Read the model definition and answer for the solid it produces. Units are mm, in the model's axes. Face numbers are marked on the shaded views. A direction names the side the tool comes from. Coordinates: 2 decimals unless noted, no trailing zeros. Write each loop counter-clockwise with the first axis right and the second up, starting at its lowest first coordinate (ties: lowest second). Pieces come first, ordered by that corner, then holes. Notation, with made-up numbers: M -8,-23.5 L 5,-23.5 A21 cw 5,-19.5 Z; hole C -5,2 d10. An arc over 180 degrees is marked long. Use a Markdown table: item, result. Add a question column.
from build123d import *

# Parameters (mm, degrees)
SKETCH1_W           = 168
SKETCH1_H           = 22
BOSS_EXTRUDE1_DEPTH = 17.8
SKETCH8_R           = 2
CUT_EXTRUDE4_DEPTH  = 22
CUT_EXTRUDE2_REACH  = 88.567
SKETCH5_W           = 117
SKETCH5_H           = 6
CUT_EXTRUDE3_DEPTH  = 15.8
BOSS_EXTRUDE3_REACH = 90.164
SKETCH7_W           = 47
SKETCH7_H           = 2


with BuildPart() as part:
    # Sketch1 → Boss-Extrude1 (new body)
    with BuildSketch(Plane(origin=(0, 0, 0), x_dir=(1, 0, 0), z_dir=(0, 1, 0))):
        Rectangle(SKETCH1_W, SKETCH1_H)
    extrude(amount=-BOSS_EXTRUDE1_DEPTH)

    # Sketch8 → Cut-Extrude4 (cut)
    with BuildSketch(Plane.XY.offset(11)):
        with Locations((75.8, -13.35)):
            Circle(SKETCH8_R)
    extrude(amount=-CUT_EXTRUDE4_DEPTH, mode=Mode.SUBTRACT)

    # Cut-Extrude2: up to this face of the body (flat: up to its plane)
    cut_extrude2_end = Plane(part.part.faces().sort_by_distance((0, -17.8, 0))[0])
    # Sketch5 → Cut-Extrude2 (cut, up to the picked face)
    with BuildSketch(Plane(origin=(0, 0, 0), x_dir=(1, 0, 0), z_dir=(0, 1, 0)), mode=Mode.PRIVATE) as cut_extrude2_sk1:
        with Locations((25.5, 8)):
            Rectangle(SKETCH5_W, SKETCH5_H)
    cut_extrude2_tool1 = split(extrude(cut_extrude2_sk1.sketch, amount=-CUT_EXTRUDE2_REACH, mode=Mode.PRIVATE), bisect_by=cut_extrude2_end, keep=Keep.BOTH, mode=Mode.PRIVATE)
    # Sketch5 → Cut-Extrude2 (cut, up to the picked face)
    with BuildSketch(Plane(origin=(0, 0, 0), x_dir=(1, 0, 0), z_dir=(0, 1, 0)), mode=Mode.PRIVATE) as cut_extrude2_sk2:
        with Locations((25.5, -8)):
            Rectangle(SKETCH5_W, SKETCH5_H)
    cut_extrude2_tool2 = split(extrude(cut_extrude2_sk2.sketch, amount=-CUT_EXTRUDE2_REACH, mode=Mode.PRIVATE), bisect_by=cut_extrude2_end, keep=Keep.BOTH, mode=Mode.PRIVATE)
    add(cut_extrude2_tool1.solids().sort_by(Axis((25.5, 0, -8), (0, -1, 0)))[0], mode=Mode.SUBTRACT)
    add(cut_extrude2_tool2.solids().sort_by(Axis((25.5, 0, 8), (0, -1, 0)))[0], mode=Mode.SUBTRACT)

    # Sketch6 → Cut-Extrude3 (cut)
    with BuildSketch(Plane.XZ.offset(17.8)):
        Polygon((-82, 9), (-82, -9), (-35, -9), (-35, -3), (82, -3), (82, 3), (-35, 3), (-35, 9), align=None)
    extrude(amount=-CUT_EXTRUDE3_DEPTH, mode=Mode.SUBTRACT)

    # Boss-Extrude3: up to this face of the body (flat: up to its plane)
    boss_extrude3_end = Plane(part.part.faces().sort_by_distance((-58.5, -9.9, 9))[0])
    # Sketch7 → Boss-Extrude3 (add, up to the picked face)
    with BuildSketch(Plane.XY.offset(-9), mode=Mode.PRIVATE) as boss_extrude3_sk1:
        with Locations((-58.5, -13.3)):
            Rectangle(SKETCH7_W, SKETCH7_H)
    boss_extrude3_tool1 = split(extrude(boss_extrude3_sk1.sketch, amount=BOSS_EXTRUDE3_REACH, mode=Mode.PRIVATE), bisect_by=boss_extrude3_end, keep=Keep.BOTH, mode=Mode.PRIVATE)
    add(boss_extrude3_tool1.solids().sort_by(Axis((-58.5, -13.3, -9), (0, 0, 1)))[0])


solid = part.part
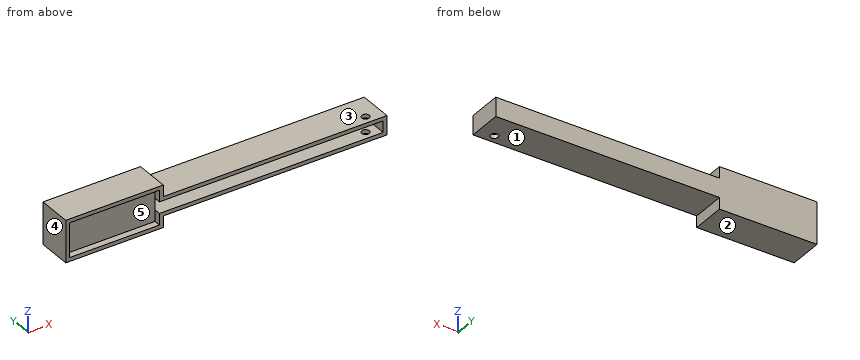
Item 1: Find section B-B on x = 75.8. Give the vertices of the cut face in (y, z).
Item 2: Find section C-C on z = -1.25. Give the vertices of the cut face in (x, y).
Item 3: Find section D-D on x = -44. Give the vertices of the cut face in (y, z).
Item 4: Consider probe 1 along Z at (x, y) = (-39, -11.25); probe 2 along Y at (x, z) = (-74, 3); probe 3 along Y at (x, z) = (75.8, -3.8). Determine where each line is inside the solid, lowest interval first.
Item 5: Determine the mould class of the marked faces 3, 4 and 5 for opening direction X: pulls with the +X half, pulls with the -X half, needs draft (parallel to the pull), parting line crosses it, or undercut.
Item 6: Each of these flat-tipped pins is pushed along its axis until it touches: pin 1 (4.5 mm diameter, centred on x = 1, y = -10, fed in from +Z); pin 2 (9 mm diameter, centred on x = -59, z = -3.5, fed in from -Y). Where does it stop, or does it pass through?
Item 7: For the marked faces 1 and 2, determine the directions among +Z, -Z, +X, -X, +Y, -Y from which every point of the face is accessible in a straight line to the end or side of a thin tool.
Item 8: Find section A-A on y = -7. Give the vertices of the cut face in (x, z).
Geometry says:
| question | item | result |
|---|---|---|
| 1 | outline | M -17.8,-5 L -15.35,-5 L -15.35,-3 L -17.8,-3 Z; M -17.8,3 L -15.35,3 L -15.35,5 L -17.8,5 Z; M -11.35,-5 L 0,-5 L 0,5 L -11.35,5 L -11.35,3 L -2,3 L -2,-3 L -11.35,-3 Z |
| 2 | outline | M -84,-17.8 L -82,-17.8 L -82,-14.3 L -35,-14.3 L -35,-12.3 L -82,-12.3 L -82,-2 L 82,-2 L 82,-17.8 L 84,-17.8 L 84,0 L -84,0 Z |
| 3 | outline | M -17.8,-11 L 0,-11 L 0,11 L -17.8,11 L -17.8,9 L -14.3,9 L -14.3,-9 L -17.8,-9 Z; hole M -12.3,-9 L -2,-9 L -2,9 L -12.3,9 Z |
| 4 | probe 1 | z = -11 to -9, 9 to 11 |
| 4 | probe 2 | y = -14.3 to -12.3, -2 to 0 |
| 4 | probe 3 | y = -17.8 to -15.35, -11.35 to 0 |
| 5 | face 3 | needs draft |
| 5 | face 4 | pulls with the -X half |
| 5 | face 5 | undercut |
| 6 | pin 1 | stops at z = 5 |
| 6 | pin 2 | stops at y = -14.3 |
| 7 | face 1 | -Z, +X, +Y, -Y |
| 7 | face 2 | -Z, +X, -X, +Y, -Y |
| 8 | outline | M -84,-11 L -33,-11 L -33,-5 L 84,-5 L 84,5 L -33,5 L -33,11 L -84,11 Z; hole M -82,-9 L -35,-9 L -35,-3 L 82,-3 L 82,3 L -35,3 L -35,9 L -82,9 Z |
